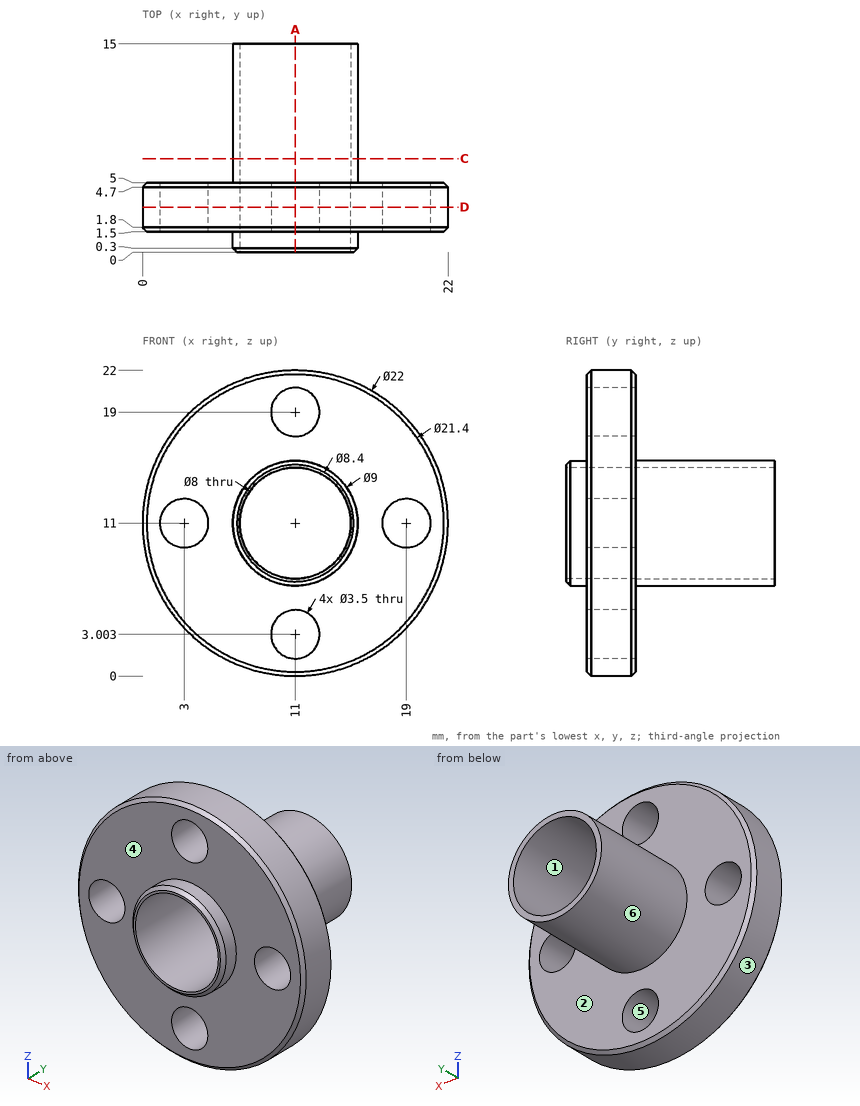
Part print with two shaded views. Sizes in mm from the minimum x, y, z corner. A direction names the side the tool comes from. Round coordinates to 2 decimals unless told otherwise and drop trailing zeros. Loops run counter-clockwise (first coordinate to the right, second up) from the corner with the lowest first, then second, coordinate; pieces in that order, holes last.
Item 1: Saw through at D-D (y = 3.25). List the corners of the cut face in (x, z).
Item 2: Drill centre lines: line 1 along Z through (x, y) = (11, 3.35); line 2 along Y through (x, z) = (16.5, 13.75); line 3 along Z through (x, y) = (9, 14.5) (1 decimal). Where is each one in solid material? Low to high.
Item 3: Saw through at C-C (y = 6.75). List the corners of the cut face in (x, z).
Item 4: Two-plate mould, pull along X, no slides. Class the marked faces 1, 2 and 3: released by +X, released by -X, zero draft, split by the parting line, or undercut.
Item 5: Saw through at A-A (x = 11). State how many separate pieces and enclosed holes the cut face has.
Item 6: Which spindle directions (+Z, -Z, +X, -X, +Y, -Y) get a long thin tool onto all of the face, cutting with end or side? Do the marked faces 4, 5 and 6. Say none if no direction does.
Item 7: Pin check, flat tips, straight feed: P1, Ø3, axis at x = 18.5, y = 8.5, coming from the -Z side; P2, Ø5.5, axis at x = 3, z = 11, coming from the -Y side; P3, Ø2, axis at y = 10, z = 13.5, coming from the -X side; P4, Ø6, axis at y = 2.5, z = 17, coming from the +X side. Stop position of each tip, or through.
Worked answers:
1. outline: circle Ø22 at (11, 11); hole circle Ø3.5 at (3, 11); hole circle Ø8 at (11, 11); hole circle Ø3.5 at (11, 3); hole circle Ø3.5 at (11, 19); hole circle Ø3.5 at (19, 11)
2. line 1: z = 0 to 1.25, 4.75 to 7, 15 to 17.25, 20.75 to 22
2. line 2: y = 1.5 to 5
2. line 3: z = 7 to 7.5, 14.5 to 15
3. outline: circle Ø9 at (11, 11); hole circle Ø8 at (11, 11)
4. face 1: undercut
4. face 2: zero draft
4. face 3: split by the parting line
5. separate pieces: 4
5. enclosed holes: 0
6. face 4: -Y
6. face 5: +Y, -Y
6. face 6: +Y
7. P1: passes through
7. P2: stops at y = 1.5
7. P3: stops at x = 6.76
7. P4: stops at x = 21.58
